```python
from build123d import *

# Parameters (mm, degrees)
F0_R            = 95.25
F0_R_2          = 14.1605
F1_DEPTH        = 3.175
F2_R            = 2.3622
F3_DEPTH        = 3.176
F3_COPIES_COUNT = 6


# Not quite as in the source:
# - a pattern or mirror of a feature is missing from the dataset's text; its kind, count and spacing are read off the source's solid


with BuildPart() as f1:
    # F0 (on Top) → F1 (new body)
    with BuildSketch(Plane.XY):
        Circle(F0_R)
        Circle(F0_R_2, mode=Mode.SUBTRACT)
    extrude(amount=F1_DEPTH)

    # F2 (on face) → F3 (cut, through all)
    with BuildSketch(Plane.XY.offset(3.175)):
        with Locations((0, 23.8125)):
            Circle(F2_R)
        with Locations((0, 76.2)):
            Circle(F2_R)
        with Locations((25.4, 43.9940905122)):
            Circle(F2_R)
    f3 = extrude(amount=-F3_DEPTH, mode=Mode.SUBTRACT)

    # F3_copies: F3 ×6 about axis
    f3_copies_axis = Axis((0, 0, 0), (0, 0, 1))
    for i in range(1, F3_COPIES_COUNT):
        add(f3.rotate(f3_copies_axis, i * 360 / F3_COPIES_COUNT), mode=Mode.SUBTRACT)


solid = f1.part
```
The listing builds one solid part. Answer for the finished solid, in the listing's coordinates (mm). Give positions to 0.01 mm unless a question says otherwise; leave off trailing zeros. Write each loop counter-clockwise with the first axis right and the second up, starting at its lowest first coordinate (ties: lowest second). Pieces come first, ordered by that corner, then holes. Notation, with made-up numbers: (-2.75, 0) -> (2.25, 0) arc R22 cw to (2.25, 18) -> close; hole circle Ø6 at (-4, 4). An arc over 180 degrees is marked (long way). Write item = value, one per line. Start each with the question number.
1) Straight lines are drawn through the part: line 1 along Y through (x, z) = (0, 1.5); line 2 along Y through (x, z) = (-66.5, 0.3); line 3 along Y through (x, z) = (25.4, 2.15). For each, find the intervals that lie inside material, in ascending order.
2) The part is cut by section D-D, the plane y = 60. Determine the outline of the cut face in (x, z) (3 decimals), and give its area (3 significant figures).
3) Determine the mould class of faces 1 (the face through (-1.09, -74.104, 1.61)), 2 (the face through (-1, -20, 3.175)) for opening direction X: +X half, -X half, draft (parallel to the pull), parting line (faces both ways), or undercut.
4) The part is cut by section A-A, the plane x = 0. Count the separate pieces of the cut face and the enclosed holes in it, and give its area (3 significant figures).
5) This flat-tipped pin is pushed along its axis until it touches: pin 1 (1 mm diameter, centred on y = -36.5, z = 2, fed in from +X). Where does it stop, or does it pass through?
6) The part is cut by section B-B, the plane y = -76.2. Determine the outline of the cut face in (x, z) (3 decimals).
Solutions:
q1.line_1 = -95.25 to -78.56, -73.84 to -26.17, -21.45 to -14.16, 14.16 to 21.45, 26.17 to 73.84, 78.56 to 95.25
q1.line_2 = -68.19 to -40.41, -35.79 to 35.79, 40.41 to 68.19
q1.line_3 = -91.8 to -46.36, -41.63 to 41.63, 46.36 to 91.8
q2.outline = (-73.977, 0) -> (73.977, 0) -> (73.977, 3.175) -> (-73.977, 3.175) -> close
q2.area = 470 mm²
q3.face_1 = undercut
q3.face_2 = draft
q4.separate_pieces = 6
q4.enclosed_holes = 0
q4.area = 455 mm²
q5.pin_1 = 88.18
q6.outline = (-57.15, 0) -> (-2.362, 0) -> (-2.362, 3.175) -> (-57.15, 3.175) -> close; (2.362, 0) -> (57.15, 0) -> (57.15, 3.175) -> (2.362, 3.175) -> close
